Could you check a few things on this model? Use its own coordinates, in mm. A direction names the side the tool comes from. Coordinates: 2 decimals unless noted, no trailing zeros. Write each loop counter-clockwise with the first axis right and the second up, starting at its lowest first coordinate (ties: lowest second). Pieces come first, ordered by that corner, then holes.
Item 1: I want a section at C-C on z = 7.5. Please give me the cut outline in (x, y), then the cut area to 3 significant figures.
Item 2: I want a section at B-B on y = 0. Please give me the cut outline in (x, z), then the cut area to 3 significant figures.
Item 3: Which directions (+Z, -Z, +X, -X, +Y, -Y) give clear straight access to the entire face, cutting with the end or side of a thin tool? Please do faces 1 (the flat face through (2.4, 0, 16)), 2 (the cylindrical face through (-0.338, 2.578, 3.972)), 3 (the flat face through (0, 0, 2)).
Item 4: I want a section at D-D on x = -0.85. Please give me the cut outline in (y, z).
Item 5: I want a section at A-A on x = 0. Please give me the cut outline in (y, z), then the cut area to 3 significant figures.
Item 6: For P1, Ø1, axis at x = 1.5, z = 16.5, coming from the +Y side; P2, Ø1.1, axis at y = 0, z = 15, coming from the +X side; P3, Ø0.5, axis at x = 2.5, y = 0, coming from the +Z side, each with a flat end and sliding along its axis, tell me the tip position at first contact or that it passes through.
Item 7: If I drill on probe 1 along X at (y, z) = (-0.15, 8.25); probe 2 along Z at (x, y) = (-0.65, 2.7); probe 3 along Y at (x, z) = (-0.6, 19), over which ranges is the centre line in solid material (lowest first)?
from build123d import *

# Parameters (mm, degrees)
F_01_START                              = 6
S01_OUTPUT_SHAFT_R                      = 3
F_01_OUTPUT_SHAFT_DEPTH                 = 16
F_02_START                              = 10
S02_D_FLAT_ON_EXPOSED_TIP_W             = 1.6
S02_D_FLAT_ON_EXPOSED_TIP_H             = 8
F_02_D_FLAT_ON_EXPOSED_TIP_DEPTH        = 12.2
F_03_START                              = 2
S03_OUTPUT_PILOT_IN_GEARBOX_NOSE_R      = 2.6
F_03_OUTPUT_PILOT_IN_GEARBOX_NOSE_DEPTH = 4


with BuildPart() as part:
    # S01 - Output shaft → 01 - Output shaft (new body)
    with BuildSketch(Plane.XY.offset(F_01_START)):
        Circle(S01_OUTPUT_SHAFT_R)
    extrude(amount=F_01_OUTPUT_SHAFT_DEPTH)

    # S02 - D flat on exposed tip → 02 - D flat on exposed tip (cut)
    with BuildSketch(Plane.XY.offset(F_02_START)):
        with Locations((3.2, 0)):
            Rectangle(S02_D_FLAT_ON_EXPOSED_TIP_W, S02_D_FLAT_ON_EXPOSED_TIP_H)
    extrude(amount=F_02_D_FLAT_ON_EXPOSED_TIP_DEPTH, mode=Mode.SUBTRACT)

    # S03 - Output pilot in gearbox nose → 03 - Output pilot in gearbox nose (add)
    with BuildSketch(Plane.XY.offset(F_03_START)):
        Circle(S03_OUTPUT_PILOT_IN_GEARBOX_NOSE_R)
    extrude(amount=F_03_OUTPUT_PILOT_IN_GEARBOX_NOSE_DEPTH)


solid = part.part
Response values:
1. outline: circle Ø6 at (0, 0)
1. area: 28.3 mm2
2. outline: (-3, 6) - (-2.6, 6) - (-2.6, 2) - (2.6, 2) - (2.6, 6) - (3, 6) - (3, 10) - (2.4, 10) - (2.4, 22) - (-3, 22) - close
2. area: 110 mm2
3. face 1: +Z, +X, +Y, -Y
3. face 2: -Z
3. face 3: -Z, +X, -X, +Y, -Y
4. outline: (-2.88, 6) - (-2.46, 6) - (-2.46, 2) - (2.46, 2) - (2.46, 6) - (2.88, 6) - (2.88, 22) - (-2.88, 22) - close
5. outline: (-3, 6) - (-2.6, 6) - (-2.6, 2) - (2.6, 2) - (2.6, 6) - (3, 6) - (3, 22) - (-3, 22) - close
5. area: 117 mm2
6. P1: stops at y = 2.83
6. P2: stops at x = 2.4
6. P3: stops at z = 22
7. probe 1: x = -3 to 3
7. probe 2: z = 6 to 22
7. probe 3: y = -2.94 to 2.94
